Here's how the part is built. I have some questions about the finished solid (model axes, mm). A direction names the side the tool comes from. Round coordinates to 2 decimals unless told otherwise and drop trailing zeros. Write each loop counter-clockwise with the first axis right and the second up, starting at its lowest first coordinate (ties: lowest second). Pieces come first, ordered by that corner, then holes. Notation, with made-up numbers: (79.5, 70) - (111.5, 70) arc R16 cw to (111.5, 98) - close; hole circle Ø6 at (-14.75, 19.25). An arc over 180 degrees is marked (long way). One line per item, written item: value. Start each with the question number.
Item 1: Imagine slicing it at D-D, the plane y = 4. Please give me the cut outline in (x, z), then the cut area to 3 significant figures.
Item 2: Imagine slicing it at B-B, the plane x = 3.75. Please give me the cut outline in (y, z), then the cut area to 3 significant figures.
Item 3: For faces 1 (the face through (5, 5, 0)), 2 (the face through (15, 6, -2)), 3 (the face through (16, 2, 2)), which set-ups out of +Z, -Z, +X, -X, +Y, -Y let a thin tool reach every point of the face, with its end or its side?
Item 4: For P1, Ø8, axis at y = 2.5, z = 0, coming from the -X side; P2, Ø4, axis at y = 0, z = 0, coming from the +X side; P3, Ø2, axis at x = 3.5, y = 1.5, coming from the -Z side; P4, Ø2, axis at x = 3.75, y = 0, coming from the +Z side, each with a flat end and sliding along its axis, tell me the tip position at first contact or that it passes through.
Item 5: Imagine slicing it at C-C, the plane z = 2.75. Please give me the cut outline in (x, y).
Item 6: Thinking about a two-plate mould opening in X: for faces 4 (the face through (0, -2, 2)), 5 (the face through (5, 0, 5)), 6 (the face through (15.51, 7.81, 1.73)), which applies, released by +X, released by -X, zero draft, split by the parting line, or undercut?
Item 7: If I drill on line 1 (X direction, y = 7.25, z = 2); line 2 (X direction, y = 4.6, z = 0); line 3 (X direction, y = 0, z = 6.3), over which ranges is the centre line in solid material (lowest first)?
Item 8: Imagine slicing it at A-A, the plane y = -6.5. Please give me the cut outline in (x, z).
```python
from build123d import *

# Parameters (mm, degrees)
SKETCH2_W = 1.25
SKETCH2_H = 8
SKETCH4_W = 1.25
SKETCH4_H = 8


with BuildPart() as part:
    # Sketch1 → Revolve1 (revolve)
    with BuildSketch(Plane.XY, mode=Mode.PRIVATE) as revolve1_sk:
        Polygon((0, 2.5), (0, 8), (7.5, 8), (7.5, 6.1), (15, 6.1), (15, 8), (16, 8), (16, 2.5), align=None)
    revolve(revolve1_sk.sketch.rotate(Axis((0, 0, 0), (-1, 0, 0)), 90), axis=Axis((0, 0, 0), (-1, 0, 0)))

    # Sketch2 → M3x0.5 Tapped Hole1 (revolve, cut)
    with BuildSketch(Plane(origin=(3.75, 0, 0), x_dir=(0, 0, -1), z_dir=(1, 0, 0))):
        with Locations((0.625, 4)):
            Rectangle(SKETCH2_W, SKETCH2_H)
    revolve(axis=Axis((3.75, -6.35, 0), (0, 1, 0)), mode=Mode.SUBTRACT)

    # Sketch4 → M3x0.5 Tapped Hole2 (revolve, cut)
    with BuildSketch(Plane.YZ.offset(3.75)):
        with Locations((0.625, 4)):
            Rectangle(SKETCH4_W, SKETCH4_H)
    revolve(axis=Axis((3.75, 0, -6.35), (0, 0, 1)), mode=Mode.SUBTRACT)


solid = part.part
```
Values follow:
1. outline: (0, -6.93) - (7.5, -6.93) - (7.5, -4.61) - (15, -4.61) - (15, -6.93) - (16, -6.93) - (16, 6.93) - (15, 6.93) - (15, 4.61) - (7.5, 4.61) - (7.5, 6.93) - (0, 6.93) - close; hole circle Ø2.5 at (3.75, 0)
1. area: 182 mm^2
2. outline: (-1.25, 2.17) - (-1.25, 7.9) arc R8 ccw (long way) to (7.9, -1.25) - (2.17, -1.25) arc R2.5 cw (long way) to start; (1.25, 2.17) arc R2.5 cw to (2.17, 1.25) - (7.9, 1.25) arc R8 ccw to (1.25, 7.9) - close
2. area: 154 mm^2
3. face 1: +Y
3. face 2: none
3. face 3: +Z, -Z, +X, +Y, -Y
4. P1: stops at x = 0
4. P2: passes through
4. P3: stops at z = -7.98
4. P4: stops at z = -2.29
5. outline: (0, -7.51) - (7.5, -7.51) - (7.5, -5.44) - (15, -5.44) - (15, -7.51) - (16, -7.51) - (16, 7.51) - (15, 7.51) - (15, 5.44) - (7.5, 5.44) - (7.5, 7.51) - (0, 7.51) - close; hole circle Ø2.5 at (3.75, 0)
6. face 4: released by -X
6. face 5: undercut
6. face 6: zero draft
7. line 1: x = 0 to 7.5, 15 to 16
7. line 2: x = 0 to 2.5, 5 to 16
7. line 3: x = 0 to 2.5, 5 to 7.5, 15 to 16
8. outline: (0, -4.66) - (7.5, -4.66) - (7.5, 4.66) - (0, 4.66) - close; (15, -4.66) - (16, -4.66) - (16, 4.66) - (15, 4.66) - close
